Can you work these out from the model? Positions are in its coordinate system, mm. A direction names the side the tool comes from. Give positions to 0.01 mm unless a question says otherwise; leave off trailing zeros. Order: outer loops, then holes, each group sorted by start corner. A loop starts at its lowest first (then second) coordinate and runs counter-clockwise, first axis right, second up. Notation, with made-up numbers: (-7, 23) -> (5, 23) arc R9 ccw to (5, 36) -> close; hole circle Ø9 at (75.5, 23.5). An arc over 180 degrees is marked (long way). Answer as CSV lines item,"result".
```python
from build123d import *

# Parameters (mm, degrees)
BOSS_EXTRU_1_DEPTH      = 0.6
ESQUISSE2_W             = 117.961397218
ESQUISSE2_H             = 91.146128779
ESQUISSE2_W_2           = 35
ESQUISSE2_H_2           = 51.049946684
ENL_V_MAT_EXTRU_1_DEPTH = 47.375774926
CONG_1_R                = 1
ENL_V_MAT_EXTRU_2_DEPTH = 26.509067015


with BuildPart() as part:
    # Esquisse1 → Boss.-Extru.1 (new body)
    with BuildSketch(Plane(origin=(0, 0, 0), x_dir=(1, 0, 0), z_dir=(0, 1, 0))):
        with BuildLine():
            Line((7, 16.35), (39.5, 16.35))
            ThreePointArc((39.5, 16.35), (41.621320344, 15.471320344), (42.5, 13.35))
            Line((42.5, 13.35), (42.5, -13.35))
            ThreePointArc((42.5, -13.35), (41.621320344, -15.471320344), (39.5, -16.35))
            Line((39.5, -16.35), (-39.5, -16.35))
            ThreePointArc((-39.5, -16.35), (-41.621320344, -15.471320344), (-42.5, -13.35))
            Line((-42.5, -13.35), (-42.5, 13.35))
            ThreePointArc((-42.5, 13.35), (-41.621320344, 15.471320344), (-39.5, 16.35))
            Line((-39.5, 16.35), (-7, 16.35))
            ThreePointArc((-7, 16.35), (-6.292893219, 16.642893219), (-6, 17.35))
            Line((-6, 17.35), (-6, 17.55))
            ThreePointArc((-6, 17.55), (-5.707106781, 18.257106781), (-5, 18.55))
            Line((-5, 18.55), (-2.3, 18.55))
            ThreePointArc((-2.3, 18.55), (-1.592893219, 18.257106781), (-1.3, 17.55))
            Line((-1.3, 17.55), (-1.3, 15.362970147))
            Line((-1.3, 15.362970147), (1.3, 15.362970147))
            Line((1.3, 15.362970147), (1.3, 17.55))
            ThreePointArc((1.3, 17.55), (1.592893219, 18.257106781), (2.3, 18.55))
            Line((2.3, 18.55), (5, 18.55))
            ThreePointArc((5, 18.55), (5.707106781, 18.257106781), (6, 17.55))
            Line((6, 17.55), (6, 17.35))
            ThreePointArc((6, 17.35), (6.292893219, 16.642893219), (7, 16.35))
        make_face()
        with BuildLine():
            Line((-3.87177285, 6.8), (3.87177285, 6.8))
            ThreePointArc((3.87177285, 6.8), (7.825, 0), (3.87177285, -6.8))
            Line((3.87177285, -6.8), (-3.87177285, -6.8))
            ThreePointArc((-3.87177285, -6.8), (-7.825, 0), (-3.87177285, 6.8))
        make_face(mode=Mode.SUBTRACT)
    extrude(amount=BOSS_EXTRU_1_DEPTH)

    # Esquisse2 → Enlèv. mat.-Extru.1 (cut, through all)
    with BuildSketch(Plane(origin=(0, 0.6, 0), x_dir=(1, 0, 0), z_dir=(0, 1, 0))):
        with Locations((-0.999168038, 1.097201222)):
            Rectangle(ESQUISSE2_W, ESQUISSE2_H)
        Rectangle(ESQUISSE2_W_2, ESQUISSE2_H_2, mode=Mode.SUBTRACT)
    extrude(amount=-ENL_V_MAT_EXTRU_1_DEPTH, mode=Mode.SUBTRACT)

    # Congé1
    cong_1_edges = [part.edges().sort_by_distance(p)[0] for p in [
        (-17.5, 0.3, -16.35),
        (17.5, 0.3, -16.35),
        (17.5, 0.3, 16.35),
        (-17.5, 0.3, 16.35),
    ]]
    fillet(cong_1_edges, radius=CONG_1_R)

    # Esquisse3 → Enlèv. mat.-Extru.2 (cut, through all)
    with BuildSketch(Plane(origin=(0, 0.6, 0), x_dir=(1, 0, 0), z_dir=(0, 1, 0))):
        with BuildLine():
            Line((-3.911281759, -6.95), (3.911281759, -6.95))
            ThreePointArc((3.911281759, -6.95), (7.975, 0), (3.911281759, 6.95))
            Line((3.911281759, 6.95), (-3.911281759, 6.95))
            ThreePointArc((-3.911281759, 6.95), (-7.975, 0), (-3.911281759, -6.95))
        make_face()
    extrude(amount=-ENL_V_MAT_EXTRU_2_DEPTH, mode=Mode.SUBTRACT)


solid = part.part
```
Item 1: We'd pull the mould along X, two halves only. Please class faces 4 (the cylindrical face through (17.215, 0.304, 16.049)), 5 (the cylindrical face through (1.585, 0.296, -18.249)), 6 (the cylindrical face through (-17.199, 0.296, -16.065)): released by +X, released by -X, zero draft, split by the parting line, or undercut.
Numbers:
face 4,"released by +X"
face 5,"undercut"
face 6,"released by -X"
Item 2: Imagine slicing it at B-B, the plane z = -3.5. Please give me the cut outline in (x, y).
Numbers:
outline,"(-17.5, 0) -> (-7.17, 0) -> (-7.17, 0.6) -> (-17.5, 0.6) -> close; (7.17, 0) -> (17.5, 0) -> (17.5, 0.6) -> (7.17, 0.6) -> close"
Item 3: Imagine slicing it at C-C, the plane y = 0.15. Please give me the cut outline in (x, z) (3 decimals).
Numbers:
outline,"(-17.5, -15.35) arc R1 ccw to (-16.5, -16.35) -> (-7, -16.35) arc R1 cw to (-6, -17.35) -> (-6, -17.55) arc R1 ccw to (-5, -18.55) -> (-2.3, -18.55) arc R1 ccw to (-1.3, -17.55) -> (-1.3, -15.363) -> (1.3, -15.363) -> (1.3, -17.55) arc R1 ccw to (2.3, -18.55) -> (5, -18.55) arc R1 ccw to (6, -17.55) -> (6, -17.35) arc R1 cw to (7, -16.35) -> (16.5, -16.35) arc R1 ccw to (17.5, -15.35) -> (17.5, 15.35) arc R1 ccw to (16.5, 16.35) -> (-16.5, 16.35) arc R1 ccw to (-17.5, 15.35) -> close; hole (-3.911, -6.95) -> (3.911, -6.95) arc R7.975 ccw to (3.911, 6.95) -> (-3.911, 6.95) arc R7.975 ccw to start"
Item 4: Imagine slicing it at A-A, the plane x = -3. Please give me the cut outline in (y, z).
Numbers:
outline,"(0, -18.55) -> (0.6, -18.55) -> (0.6, -6.95) -> (0, -6.95) -> close; (0, 6.95) -> (0.6, 6.95) -> (0.6, 16.35) -> (0, 16.35) -> close"
Item 5: Please list where these lines run through material, in increasing order: line 1 along Z through (x, y) = (-12, 0.1); line 2 along Z through (x, y) = (-5, 0.15); line 3 along Z through (x, y) = (-4, 0.15).
Numbers:
line 1,"z = -16.35 to 16.35"
line 2,"z = -18.55 to -6.21, 6.21 to 16.35"
line 3,"z = -18.55 to -6.9, 6.9 to 16.35"
Item 6: For faces 1 (the cylindrical face through (-1.601, 0.296, -18.265)), 2 (the flat face through (8.02, 0.6, -1.34)), 3 (the cylindrical face through (-7.974, 0.304, -0.118)), which set-ups out of +Z, -Z, +X, -X, +Y, -Y let a thin tool reach every point of the face, with its end or its side?
Numbers:
face 1,"-Z, +Y, -Y"
face 2,"+Z, -Z, +X, -X, +Y"
face 3,"+Y, -Y"
Item 7: For pin 1 (4 mm diameter, centred on x = -11, z = 9, fed in from -Y); pin 2 (5 mm diameter, centred on x = -1.5, z = 2, fed in from +Y), each with a flat end and sliding along its axis, tell me the tip position at first contact or that it passes through.
Numbers:
pin 1,"stops at y = 0"
pin 2,"passes through"
Item 8: Imagine slicing it at D-D, the plane x = -10. Please give me the cut outline in (y, z), then the cut area to 3 significant figures.
Numbers:
outline,"(0, -16.35) -> (0.6, -16.35) -> (0.6, 16.35) -> (0, 16.35) -> close"
area,"19.6 mm²"
